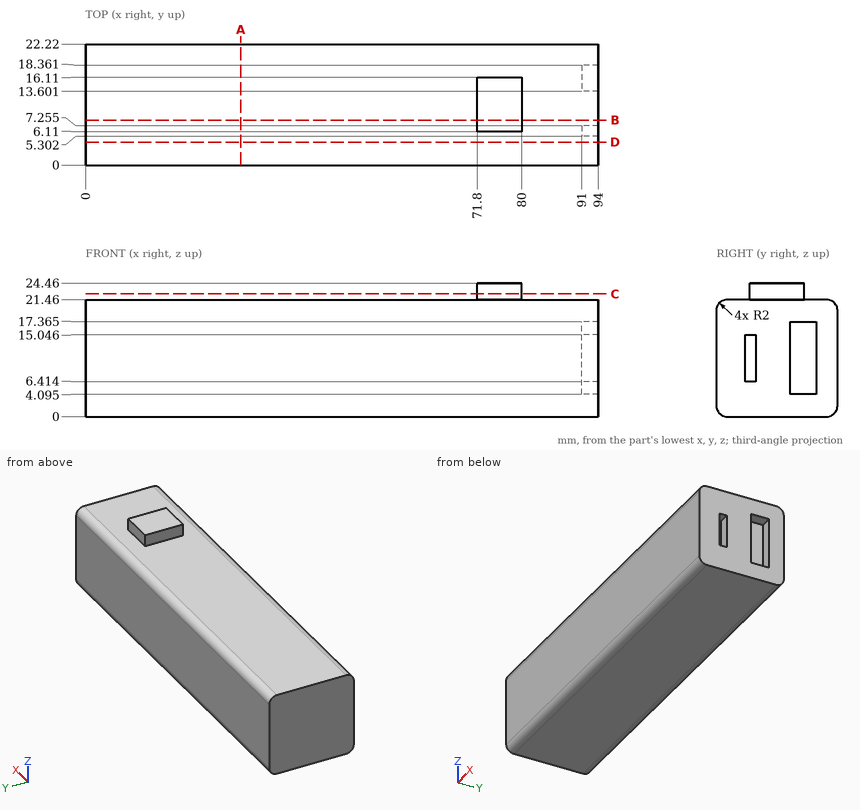
Verification items for this drawing (mm, ordinates from the low corner). Coordinates: 2 decimals unless noted, no trailing zeros. Order: outer loops, then holes, each group sorted by start corner. A loop starts at its lowest first (then second) coordinate and runs counter-clockwise, first axis right, second up. Notation, with made-up numbers: M -37.5,-15.75 L 4.5,-15.75 A3 cw 4.5,-11.75 Z; hole C 15.5,21 d7. An arc over 180 degrees is marked long. One line per item, written item: value. Start each with the question number.
Item 1: Thickness scan on probe 1 along Z at (x, y) = (36, 16.75); probe 2 along X at (y, z) = (15, 10.5); probe 3 along Y at (x, z) = (6, 1.75) (1 decimal). Record the ranges inside material, lowest first.
Item 2: Sectioned sample at A-A on x = 28.5. Record the cut outline in (y, z), then the cut area to 3 significant figures.
Item 3: Sectioned sample at B-B on y = 8.25. Record the cut outline in (x, z), then the cut area to 3 significant figures.
Item 4: Depth check by flat-ended pin: P1, Ø1, axis at y = 17.5, z = 9, coming from the +X side; P2, Ø0.9, axis at x = 76, z = 23, coming from the -Y side; P3, Ø8, axis at x = 37, y = 13, coming from the +Z side. Enter the tip coordinate at first touch or a pass-through.
Item 5: Sectioned sample at D-D on y = 4.25. Record the cut outline in (x, z), then the cut area to 3 significant figures.
Item 6: Sectioned sample at C-C on z = 22.5. Record the cut outline in (x, y), then the cut area to 3 significant figures.
Calculated:
1. probe 1: 0 to 21.46
1. probe 2: 0 to 91
1. probe 3: 0 to 22.2
2. outline: M 0,2 A2 ccw 2,0 L 20.22,0 A2 ccw 22.22,2 L 22.22,19.46 A2 ccw 20.22,21.46 L 2,21.46 A2 ccw 0,19.46 Z
2. area: 473 mm^2
3. outline: M 0,0 L 94,0 L 94,21.46 L 80,21.46 L 80,24.46 L 71.8,24.46 L 71.8,21.46 L 0,21.46 Z
3. area: 2,040 mm^2
4. P1: x = 91
4. P2: y = 6.11
4. P3: z = 21.46
5. outline: M 0,0 L 94,0 L 94,21.46 L 0,21.46 Z
5. area: 2,020 mm^2
6. outline: M 71.8,6.11 L 80,6.11 L 80,16.11 L 71.8,16.11 Z
6. area: 82.0 mm^2
